For this review, take the finished solid that the model builds, in its own axes (mm). A direction names the side the tool comes from. Coordinates: 2 decimals unless noted, no trailing zeros. Write each loop counter-clockwise with the first axis right and the second up, starting at its lowest first coordinate (ties: lowest second). Pieces come first, ordered by that corner, then holes.
1) We need section B-B on y = 2.5. Write out the cut boundary in (x, z).
2) We need section C-C on z = -5.75. Write out the cut boundary in (x, y), then the cut area to 3 significant figures.
3) Insertion check: P1, Ø6, axis at x = 7, z = -7, coming from the +Y side; P2, Ø0.6, axis at x = -9.5, y = 48.5, coming from the +Z side; P3, Ø1.6, axis at x = 0, z = -1, coming from the +Y side. Each pin has a flat end and moves straight along its axis. Give the tip position at first contact, or say it passes through.
4) To check wall thickness, follow line 1 along X through (y, z) = (28.5, -16); line 2 along Z through (x, y) = (6, 15.5); line 3 along X through (y, z) = (-6, -1). State the ranges of each line that lie inside material, in increasing order.
5) For faces 4 (the face through (9.237, 8, -11)), 5 (the face through (0, -46.461, -0.4)), list the 3-axis set-ups (+Z, -Z, +X, -X, +Y, -Y) from which the entire face can be reached by the end or side of a thin tool; tool diameter is ignored.
6) Mouldability with a two-part tool opening along Z and no side actions: class faces 1 (the face through (-9.973, 8, -11)), 2 (the face through (-9.6, 50.8, -13.1)), 3 (the face through (0, -1, 0)) as pulls with the +Z half, pulls with the -Z half, needs draft (parallel to the pull), parting line crosses it, or undercut.
7) We need section A-A on z = -15. Write out the cut boundary in (x, y).
8) We need section D-D on x = -6.5. Write out the cut boundary in (y, z).
from build123d import *

# Parameters (mm, degrees)
SKETCH1_W               = 15
SKETCH1_H               = 92.922077922
BASE_FLANGE1_DEPTH      = 0.7366
EDGE_FLANGE2_DEPTH      = 92.922077922
EDGE_FLANGE2_BEND_DEPTH = 92.922077922
SKETCH31_R              = 2.1
TAB3_DEPTH              = 0.7366
TAB4_START              = -0.7366
SKETCH35_R              = 2.1
TAB4_DEPTH              = 0.7366


# Sheet-metal steps are written as plain solids
with BuildPart() as part:
    # Sketch1 → Base-Flange1 (new body)
    with BuildSketch(Plane.XY):
        Rectangle(SKETCH1_W, SKETCH1_H)
    extrude(amount=-BASE_FLANGE1_DEPTH)

    # Edge-Flange2 section (across the edge) → Edge-Flange2 (add)
    with BuildSketch(Plane(origin=(9.2366, 46.461038961, -0.7366), x_dir=(-1, 0, 0), z_dir=(0, -1, 0))):
        with BuildLine():
            Line((-0.7366, 0.7366), (-0.7366, 20))
            Line((-0.7366, 20), (0, 20))
            Line((0, 20), (0, 0.7366))
            ThreePointArc((0, 0.7366), (0.215745145, 0.215745145), (0.7366, 0))
            Line((0.7366, 0), (1.7366, 0))
            Line((1.7366, 0), (1.7366, -0.7366))
            Line((1.7366, -0.7366), (0.7366, -0.7366))
            ThreePointArc((0.7366, -0.7366), (-0.30510971, -0.30510971), (-0.7366, 0.7366))
        make_face()
    extrude(amount=EDGE_FLANGE2_DEPTH)

    # Edge-Flange2 section 2 (across the edge) → Edge-Flange2 bend (add)
    with BuildSketch(Plane(origin=(-9.2366, -46.461038961, -0.7366), x_dir=(1, 0, 0), z_dir=(0, 1, 0))):
        with BuildLine():
            Line((-0.7366, 0.7366), (-0.7366, 20))
            Line((-0.7366, 20), (0, 20))
            Line((0, 20), (0, 0.7366))
            ThreePointArc((0, 0.7366), (0.215745145, 0.215745145), (0.7366, 0))
            Line((0.7366, 0), (1.7366, 0))
            Line((1.7366, 0), (1.7366, -0.7366))
            Line((1.7366, -0.7366), (0.7366, -0.7366))
            ThreePointArc((0.7366, -0.7366), (-0.30510971, -0.30510971), (-0.7366, 0.7366))
        make_face()
    extrude(amount=EDGE_FLANGE2_BEND_DEPTH)

    # Sketch31 → Tab3 (add)
    with BuildSketch(Plane(origin=(9.9732, 0, 0), x_dir=(0, 0, -1), z_dir=(1, 0, 0))):
        with BuildLine():
            Line((1.4732, 46.461038961), (1.4732, 51.461038961))
            ThreePointArc((1.4732, 51.461038961), (11.1049, 61.092738961), (20.7366, 51.461038961))
            Line((20.7366, 51.461038961), (20.7366, 46.461038961))
            Line((20.7366, 46.461038961), (1.4732, 46.461038961))
        make_face()
        with Locations((11.1049, 51.461038961)):
            Circle(SKETCH31_R, mode=Mode.SUBTRACT)
    extrude(amount=-TAB3_DEPTH)

    # Sketch35 → Tab4 (add)
    with BuildSketch(Plane.ZY.offset(9.9732).offset(TAB4_START)):
        with BuildLine():
            Line((-20.7366, 46.461038961), (-20.7366, 51.461038961))
            ThreePointArc((-20.7366, 51.461038961), (-11.1049, 61.092738961), (-1.4732, 51.461038961))
            Line((-1.4732, 51.461038961), (-1.4732, 46.461038961))
            Line((-1.4732, 46.461038961), (-20.7366, 46.461038961))
        make_face()
        with Locations(Location((-11.1049, 51.461038961, 0), (0, 0, 180))):
            Circle(SKETCH35_R, mode=Mode.SUBTRACT)
    extrude(amount=TAB4_DEPTH)


solid = part.part
Result:
1. outline: (-9.97, -20.74) - (-9.24, -20.74) - (-9.24, -1.47) arc R0.74 cw to (-8.5, -0.74) - (8.5, -0.74) arc R0.74 cw to (9.24, -1.47) - (9.24, -20.74) - (9.97, -20.74) - (9.97, -1.47) arc R1.47 ccw to (8.5, 0) - (-8.5, 0) arc R1.47 ccw to (-9.97, -1.47) - close
2. outline: (-9.97, -46.46) - (-9.24, -46.46) - (-9.24, 59.47) - (-9.97, 59.47) - close; (9.24, -46.46) - (9.97, -46.46) - (9.97, 59.47) - (9.24, 59.47) - close
2. area: 156 mm2
3. P1: stops at y = 60.86
3. P2: stops at z = -1.47
3. P3: stops at y = 46.46
4. line 1: x = -9.97 to -9.24, 9.24 to 9.97
4. line 2: z = -0.74 to 0
4. line 3: x = -9.9 to -9.06, 9.06 to 9.9
5. face 4: -Z, +Y, -Y
5. face 5: +Z, -Z, +X, -X, -Y
6. face 1: needs draft
6. face 2: undercut
6. face 3: pulls with the +Z half
7. outline: (-9.97, -46.46) - (-9.24, -46.46) - (-9.24, 60.27) - (-9.97, 60.27) - close; (9.24, -46.46) - (9.97, -46.46) - (9.97, 60.27) - (9.24, 60.27) - close
8. outline: (-46.46, -0.74) - (46.46, -0.74) - (46.46, 0) - (-46.46, 0) - close
